Design review of the part built by this model. Coordinates are the model's own, in mm. Face numbers are marked on the shaded views. Coordinates: 2 decimals unless noted, no trailing zeros. Loops run counter-clockwise (first coordinate to the right, second up) from the corner with the lowest first, then second, coordinate; pieces in that order, holes last. Notation, with made-up numbers: (83.5, 51.25) - (110.5, 51.25) arc R19 ccw to (110.5, 84.25) - close; hole circle Ø1 at (75.5, -7.5). An arc over 180 degrees is marked (long way). Return JSON: item names as keys, results as strings. Group by question number.
Autodesk Inventor part; units mm, degrees
ref_plane "YZ Plane" through (0, 0, 0) normal (1, 0, 0) x (0, 1, 0)
ref_plane "XZ Plane" through (0, 0, 0) normal (0, 1, 0) x (-1, 0, 0)
ref_plane "XY Plane" through (0, 0, 0) normal (0, 0, 1) x (1, 0, 0)
sketch "Skizze1" plane through (0, 0, 0) normal (0, 0, 1) x (1, 0, 0)
  arc A0 (-47.2504, 56.6131) -> (-53.0963, 48.2064) centre (-45.1265, 48.9002) ccw
  arc A1 (47.2504, 56.6131) -> (-47.2504, 56.6131) centre (0, -114.9743) ccw
  arc A2 (53.0963, 48.2064) -> (47.2504, 56.6131) centre (45.1265, 48.9002) ccw
  line L0 (53.0963, 48.2064) -> (44.103, -55.104)
  arc A3 (38.7321, -61.9763) -> (44.103, -55.104) centre (36.1331, -54.4103) ccw
  arc A4 (-38.7321, -61.9763) -> (38.7321, -61.9763) centre (0, 50.7799) ccw
  arc A5 (-44.103, -55.104) -> (-38.7321, -61.9763) centre (-36.1331, -54.4103) ccw
  line L1 (-44.103, -55.104) -> (-53.0963, 48.2064)
  circle A6 centre (0, -62.4432) radius 1.6
  circle A7 centre (0, 57) radius 1.6
  circle A8 centre (-44.9364, 46.717) radius 2.1
  circle A9 centre (-36.329, -52.1602) radius 2.1
  circle A10 centre (0, 0) radius 2.1
  circle A11 centre (44.9364, 46.717) radius 2.1
  circle A12 centre (36.329, -52.1602) radius 2.1
  circle A13 centre (-44.9364, 46.717) radius 4
  circle A14 centre (44.9364, 46.717) radius 4
  circle A15 centre (36.329, -52.1602) radius 4
  circle A16 centre (-36.329, -52.1602) radius 4
  circle A17 centre (0, -62.4432) radius 3.5
  circle A18 centre (0, 57) radius 3.5
  circle A19 centre (0, 0) radius 20
  arc A20 (-46.1884, 52.7567) -> (-49.1114, 48.5533) centre (-45.1265, 48.9002) ccw
  line L2 (-49.1114, 48.5533) -> (-40.118, -54.7572)
  arc A21 (-40.118, -54.7572) -> (-37.4326, -58.1933) centre (-36.1331, -54.4103) ccw
  arc A22 (-37.4326, -58.1933) -> (37.4326, -58.1933) centre (0, 50.7799) ccw
  arc A23 (37.4326, -58.1933) -> (40.118, -54.7572) centre (36.1331, -54.4103) ccw
  line L3 (40.118, -54.7572) -> (49.1114, 48.5533)
  arc A24 (49.1114, 48.5533) -> (46.1884, 52.7567) centre (45.1265, 48.9002) ccw
  arc A25 (46.1884, 52.7567) -> (-46.1884, 52.7567) centre (0, -114.9743) ccw
  circle A26 centre (0, 0) radius 24
  point P0 (0, 0)
  point P1 (-2.8888, 58.976)
  point P2 (2.8888, 58.976)
  point P3 (2.8973, -64.4067)
  point P4 (-2.8973, -64.4067)
  dimension "d0" = 8
  dimension "d1" = 8
  dimension "d2" = 8
  dimension "d3" = 8
  dimension "d4" = 7
  dimension "d5" = 7
  dimension "d6" = 40
  dimension "d7" = 4
  dimension "d8" = 4
extrude "Extrusion1" add sketch "Skizze1" against normal blind 5 contours A1 A2 L0 A3 A4 A5 L1 A0 | L2 A20 A25 A18 A24 L3 A23 A22 A17 A21 | A25 A18 | A18 A25 | A22 A17 | A17 A22 | A19 | A26
sketch "Skizze2" plane through (0, 0, -5) normal (0, 0, -1) x (-1, 0, 0)
  circle A0 centre (0, 0) radius 26
  circle A1 centre (54.772, 35) radius 21
  circle A2 centre (54.772, 35) radius 21
  circle A3 centre (-54.772, 35) radius 21
  circle A4 centre (-54.772, 35) radius 21
  circle A5 centre (-35, -54.772) radius 21
  circle A6 centre (-35, -54.772) radius 21
  circle A7 centre (35, -54.772) radius 21
  circle A8 centre (35, -54.772) radius 21
  arc A9 (-44.0306, 77) -> (44.0306, 77) centre (0, 0) ccw
  line L0 (-29, 77) -> (-44.0306, 77)
  line L1 (-44.0306, 77) -> (44.0306, 77)
  circle A10 centre (44.9364, 46.717) radius 4
  circle A11 centre (-44.9364, 46.717) radius 4
  circle A12 centre (-36.329, -52.1602) radius 4
  circle A13 centre (36.329, -52.1602) radius 4
  circle A14 centre (0, -62.4432) radius 1.6
  circle A15 centre (0, 57) radius 1.6
  arc A16 (53.0963, 48.2064) -> (47.2504, 56.6131) centre (45.1265, 48.9002) ccw
  line L2 (53.0963, 48.2064) -> (44.103, -55.104)
  arc A17 (38.7321, -61.9763) -> (44.103, -55.104) centre (36.1331, -54.4103) ccw
  arc A18 (-38.7321, -61.9763) -> (38.7321, -61.9763) centre (0, 50.7799) ccw
  arc A19 (-44.103, -55.104) -> (-38.7321, -61.9763) centre (-36.1331, -54.4103) ccw
  line L3 (-44.103, -55.104) -> (-53.0963, 48.2064)
  arc A20 (-47.2504, 56.6131) -> (-53.0963, 48.2064) centre (-45.1265, 48.9002) ccw
  arc A21 (47.2504, 56.6131) -> (-47.2504, 56.6131) centre (0, -114.9743) ccw
  circle A22 centre (0, 0) radius 2.1
extrude "Extrusion3" add sketch "Skizze2" against normal blind 5 contours A1 L2 A16 | A7 A18 A17 L2 | A20 L3 A3 | A5 L3 A19 A18 | L0 L1 A9 picked at (55.8063, 25.5813) picked at (36.6001, -67.1417) picked at (-56.1388, 25.6369) picked at (-36.8762, -67.0802)
sketch "Skizze5" plane through (0, 0, 0) normal (0, 0, 1) x (1, 0, 0)
  circle A0 centre (0, 0) radius 20
  circle A1 centre (44.9364, 46.717) radius 4
  circle A2 centre (-44.9364, 46.717) radius 4
  circle A3 centre (-36.329, -52.1602) radius 4
  circle A4 centre (36.329, -52.1602) radius 4
  circle A5 centre (0, -62.4432) radius 1.6
  circle A6 centre (0, 57) radius 1.6
  arc A7 (53.0963, 48.2064) -> (47.2504, 56.6131) centre (45.1265, 48.9002) ccw
  line L0 (53.0963, 48.2064) -> (44.103, -55.104)
  arc A8 (38.7321, -61.9763) -> (44.103, -55.104) centre (36.1331, -54.4103) ccw
  arc A9 (-38.7321, -61.9763) -> (38.7321, -61.9763) centre (0, 50.7799) ccw
  arc A10 (-44.103, -55.104) -> (-38.7321, -61.9763) centre (-36.1331, -54.4103) ccw
  line L1 (-44.103, -55.104) -> (-53.0963, 48.2064)
  arc A11 (-47.2504, 56.6131) -> (-53.0963, 48.2064) centre (-45.1265, 48.9002) ccw
  arc A12 (47.2504, 56.6131) -> (-47.2504, 56.6131) centre (0, -114.9743) ccw
  arc A13 (-47.3832, 57.0952) -> (-53.5945, 48.1631) centre (-45.1265, 48.9002) ccw
  line L2 (-53.5945, 48.1631) -> (-44.6011, -55.1474)
  arc A14 (-44.6011, -55.1474) -> (-38.8945, -62.4492) centre (-36.1331, -54.4103) ccw
  arc A15 (-38.8945, -62.4492) -> (38.8945, -62.4492) centre (0, 50.7799) ccw
  arc A16 (38.8945, -62.4492) -> (44.6011, -55.1474) centre (36.1331, -54.4103) ccw
  line L3 (44.6011, -55.1474) -> (53.5945, 48.1631)
  arc A17 (53.5945, 48.1631) -> (47.3832, 57.0952) centre (45.1265, 48.9002) ccw
  arc A18 (47.3832, 57.0952) -> (-47.3832, 57.0952) centre (0, -114.9743) ccw
  dimension "d19" = 0.5
extrude "Extrusion5" cut sketch "Skizze5" against normal blind 2 contours A0 | A1 | A2 | A3 | A4 | A5 | A6 | L0 A8 A9 A10 L1 A11 A12 A7 | A18 A17 L3 A16 A15 A14 L2 A13
sketch "Skizze6" plane through (0, 0, -5) normal (0, 0, -1) x (-1, 0, 0)
  arc A0 (-44.0306, 77) -> (44.0306, 77) centre (0, 0) ccw
  line L0 (-44.0306, 77) -> (44.0306, 77)
  circle A1 centre (44.9364, 46.717) radius 4
  circle A2 centre (-44.9364, 46.717) radius 4
  circle A3 centre (-36.329, -52.1602) radius 4
  circle A4 centre (36.329, -52.1602) radius 4
  circle A5 centre (0, -62.4432) radius 1.6
  circle A6 centre (0, 57) radius 1.6
  circle A7 centre (0, 0) radius 2.1
  circle A8 centre (36.329, -52.1602) radius 7.5
  circle A9 centre (-36.329, -52.1602) radius 7.5
  circle A10 centre (-44.9364, 46.717) radius 7.5
  circle A11 centre (44.9364, 46.717) radius 7.5
  dimension "d37" = 15
  dimension "d38" = 15
  dimension "d39" = 15
  dimension "d40" = 15
extrude "Extrusion6" add sketch "Skizze6" along normal blind 4 contours L0 A0 | A7
sketch "Skizze7" plane through (0, 0, -9) normal (0, 0, -1) x (-1, 0, 0)
  circle A0 centre (0, 0) radius 4
  circle A1 centre (0, 0) radius 20
  circle A2 centre (0, 0) radius 2.1
  dimension "d24" = 8
  dimension "d31" = 4.2
sketch "Skizze8" plane through (0, 0, -2) normal (0, 0, 1) x (1, 0, 0)
  circle A0 centre (-44.9364, 46.717) radius 4
  circle A1 centre (-44.9364, 46.717) radius 4
  circle A2 centre (44.9364, 46.717) radius 4
  circle A3 centre (44.9364, 46.717) radius 4
  circle A4 centre (36.329, -52.1602) radius 4
  circle A5 centre (36.329, -52.1602) radius 4
  circle A6 centre (-36.329, -52.1602) radius 4
  circle A7 centre (-36.329, -52.1602) radius 4
  circle A8 centre (-44.9364, 46.717) radius 2.1
  circle A9 centre (44.9364, 46.717) radius 2.1
  circle A10 centre (36.329, -52.1602) radius 2.1
  circle A11 centre (-36.329, -52.1602) radius 2.1
  point P0 (0, 0)
  dimension "d25" = 4.2
  dimension "d26" = 4.2
  dimension "d27" = 4.2
  dimension "d28" = 4.2
extrude "Extrusion7" add sketch "Skizze8" against normal blind 1
extrude "Extrusion8" cut sketch "Skizze7" against normal up to surface (4 mm away) contours A2
sketch "Skizze9" plane through (0, 0, -2) normal (0, 0, 1) x (1, 0, 0)
  circle A0 centre (0, 0) radius 2.1
  circle A1 centre (0, 0) radius 4
  dimension "d34" = 8
extrude "Extrusion9" cut sketch "Skizze9" against normal up to surface (7 mm away) contours A0 | A1
sketch "Skizze10" plane through (-36.329, -52.1602, -5) normal (0, 0, -1) x (-1, 0, 0)
  circle A0 centre (0, 0) radius 2.1
  circle A1 centre (0, 0) radius 4
  circle A2 centre (0, 0) radius 7.5
  circle A3 centre (-72.6579, 0) radius 2.1
  circle A4 centre (-81.2654, 98.8771) radius 2.1
  circle A5 centre (8.6075, 98.8771) radius 2.1
  circle A6 centre (-72.6579, 0) radius 4
  circle A7 centre (-72.6579, 0) radius 7.5
  circle A8 centre (-81.2654, 98.8771) radius 4
  circle A9 centre (-81.2654, 98.8771) radius 7.5
  circle A10 centre (8.6075, 98.8771) radius 4
  circle A11 centre (8.6075, 98.8771) radius 7.5
  point P0 (-36.329, 52.1602)
extrude "Extrusion10" cut sketch "Skizze10" against normal up to surface (2 mm away) contours A2 | A7 | A9 | A11
fillet "Rundung2" radius 10 2 edges at (44.0306, 77, -4.5) (-44.0306, 77, -4.5)
sketch "Skizze11" plane through (0, 0, -2) normal (0, 0, 1) x (1, 0, 0)
  circle A0 centre (0, 57) radius 1.6
  circle A1 centre (0, 57) radius 2.1
  circle A2 centre (0, -62.4432) radius 1.6
  circle A3 centre (0, -62.4432) radius 2.1
  point P0 (0, 0)
  dimension "d47" = 4.2
  dimension "d48" = 4.2
extrude "Extrusion11" cut sketch "Skizze11" against normal blind 6 contours A0 | A1 | A2 | A3
sketch "Skizze12" plane through (0, 0, -9) normal (0, 0, -1) x (-1, 0, 0)
  circle A0 centre (0, -62.4432) radius 1.6
  circle A1 centre (0, -62.4432) radius 1.6
  circle A2 centre (0, 57) radius 1.6
  circle A3 centre (0, 57) radius 1.6
  point P0 (0, 0)
extrude "Extrusion12" add sketch "Skizze12" against normal up to surface (1 mm away)
chamfer "Fasen2" distance 2 angle 45 1 edges at (0, -88.7, -9)
properties part number "SpiegelabdeckungSSL"
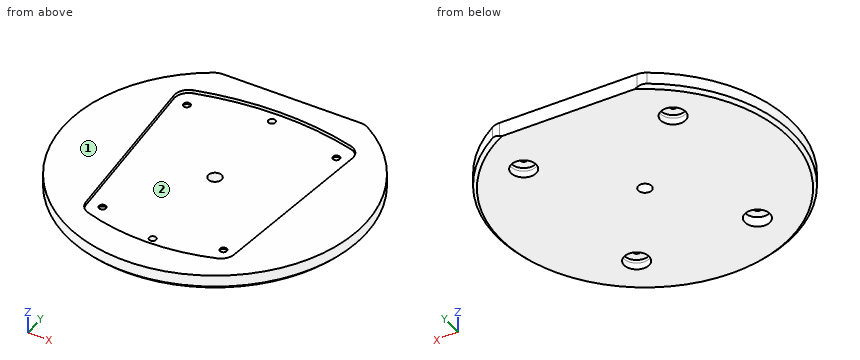
Item 1: To check wall thickness, follow line 1 (Y direction, x = 0, z = -6.1); line 2 (X direction, y = 45, z = -7.5); line 3 (Z direction, x = -43, y = 27.5). State the ranges of each line that lie inside material, in increasing order. Write a range as from..to.
Item 2: For P1, Ø9, axis at x = 44.94, y = 46.72, coming from the -Z side; P2, Ø2, axis at x = -0.5, y = 57.5, coming from the +Z side; P3, Ø2, axis at y = 4.5, z = -1.5, coming from the -X side; P4, Ø3.5, axis at x = -44.94, y = 46.72, coming from the +Z side, all flat-tipped, find the tip position at first contact; note any pin that passes through.
Item 3: Draft analysis for pull direction X (two halves, no side actions). For the marked faces 1 and 2, state which applies: pulls with the +X half, pulls with the -X half, needs draft (parallel to the pull), parting line crosses it, or undercut.
Item 4: Add section A-A (x = 0). State the section outline as (y, z) points, then the cut area to 3 significant figures.
Item 5: Add section B-B (y = 0). State the section outline as (x, z) points, then the cut area to 3 significant figures.
Answers below:
{
 "1": {"line 1": "y = -88.7..-64.54, -60.34..-4, 4..54.9, 59.1..77", "line 2": "x = -75.86..-52.24, -37.64..37.64, 52.24..75.86", "line 3": "z = -9..-2"},
 "2": {"P1": "stops at z = -3", "P2": "stops at z = -8", "P3": "stops at x = -88.63", "P4": "passes through"},
 "3": {"face 1": "needs draft", "face 2": "undercut"},
 "4": {"outline": "(-88.7, -7) - (-86.7, -9) - (-4, -9) - (-4, -2) - (-60.34, -2) - (-60.34, -8) - (-64.54, -8) - (-64.54, -2) - (-68.94, -2) - (-68.94, 0) - (-88.7, 0) - close; (4, -9) - (77, -9) - (77, 0) - (63.5, 0) - (63.5, -2) - (59.1, -2) - (59.1, -8) - (54.9, -8) - (54.9, -2) - (4, -2) - close", "area": "1,120 mm^2"},
 "5": {"outline": "(-88.7, -7) - (-86.7, -9) - (-4, -9) - (-4, -2) - (-49.4, -2) - (-49.4, 0) - (-88.7, 0) - close; (4, -9) - (86.7, -9) - (88.7, -7) - (88.7, 0) - (49.4, 0) - (49.4, -2) - (4, -2) - close", "area": "1,340 mm^2"}
}
